Geometry: see drawing. Coordinates: mm, zero at the bounding-box minimum. A direction names the side the tool comes from. Give positions to 0.01 mm unless a question says otherwise; leave off trailing zeros. Write each loop counter-clockwise with the first axis right and the second up, starting at its lowest first coordinate (ties: lowest second). Pieces come first, ordered by that corner, then holes.
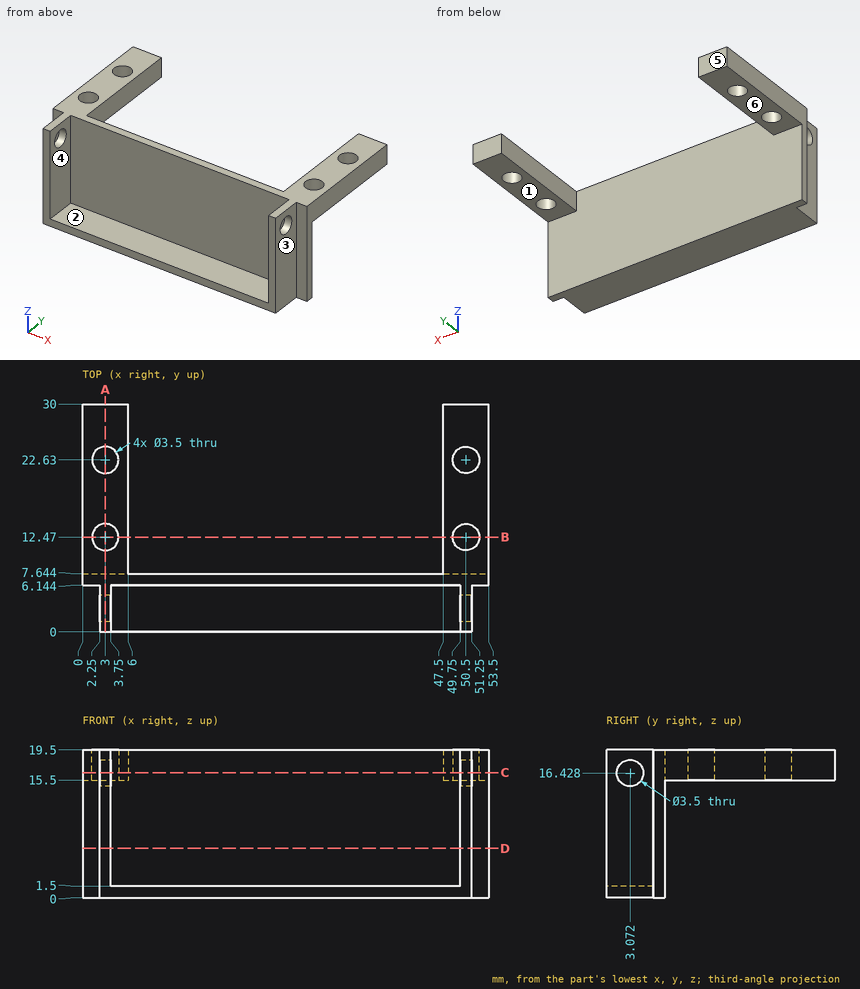
1. Pin query (flat end, axial travel): P1, Ø10, axis at x = 44.5, y = 16, coming from the -Z side; P2, Ø5, axis at y = 3, z = 10.5, coming from the +X side; P3, Ø0.7, axis at x = 52, z = 12.5, coming from the -Y side. Return the tip coordinate at first contact, or that it passes through.
2. Section query A-A (x = 3). Return loops of the section in (y, z).
3. Section query C-C (z = 16.5). Return loops of the section in (x, y).
4. Section query B-B (y = 12.47). Return loops of the section in (x, z).
5. Pull-direction query (X, two-part tool) for the marked faces 1, 2 and 3; classes: pulls with the +X half, pulls with the -X half, needs draft (parallel to the pull), parting line crosses it, or undercut.
6. Access query for the marked faces 4, 5 and 6. Directions: +Z, -Z, +X, -X, +Y, -Y. A direction counts if a zero-diameter tool reaches every point of the face in a straight line with its end or side. Return the directions, or none.
7. Line query: probe 1 along X at (y, z) = (1.5, 5); probe 2 along Y at (x, z) = (3, 17.75); probe 3 along Y at (x, z) = (3, 17.1). Output: solid intervals per line, ascending.
8. Section query D-D (z = 6.5). Return loops of the section in (x, y), plus the area to 3 significant figures.
The answers:
1. P1: stops at z = 15.5
1. P2: stops at x = 51.25
1. P3: stops at y = 6.14
2. outline: (0, 0) - (7.64, 0) - (7.64, 15.5) - (10.72, 15.5) - (10.72, 19.5) - (0, 19.5) - close; (14.22, 15.5) - (20.88, 15.5) - (20.88, 19.5) - (14.22, 19.5) - close; (24.38, 15.5) - (30, 15.5) - (30, 19.5) - (24.38, 19.5) - close; hole circle Ø3.5 at (3.07, 16.43)
3. outline: (0, 6.14) - (2.25, 6.14) - (2.25, 4.82) - (3.75, 4.82) - (3.75, 6.14) - (49.75, 6.14) - (49.75, 4.82) - (51.25, 4.82) - (51.25, 6.14) - (53.5, 6.14) - (53.5, 30) - (47.5, 30) - (47.5, 7.64) - (6, 7.64) - (6, 30) - (0, 30) - close; (2.25, 0) - (3.75, 0) - (3.75, 1.32) - (2.25, 1.32) - close; (49.75, 0) - (51.25, 0) - (51.25, 1.32) - (49.75, 1.32) - close; hole circle Ø3.5 at (3, 12.47); hole circle Ø3.5 at (3, 22.63); hole circle Ø3.5 at (50.5, 12.47); hole circle Ø3.5 at (50.5, 22.63)
4. outline: (0, 15.5) - (1.25, 15.5) - (1.25, 19.5) - (0, 19.5) - close; (4.75, 15.5) - (6, 15.5) - (6, 19.5) - (4.75, 19.5) - close; (47.5, 15.5) - (48.75, 15.5) - (48.75, 19.5) - (47.5, 19.5) - close; (52.25, 15.5) - (53.5, 15.5) - (53.5, 19.5) - (52.25, 19.5) - close
5. face 1: needs draft
5. face 2: undercut
5. face 3: pulls with the +X half
6. face 4: +Z, -Y
6. face 5: +Z, -Z, +X, -X, +Y
6. face 6: -Z, +X, -X, +Y
7. probe 1: x = 2.25 to 3.75, 49.75 to 51.25
7. probe 2: y = 0 to 1.93, 4.22 to 10.72, 14.22 to 20.88, 24.38 to 30
7. probe 3: y = 0 to 1.46, 4.69 to 10.72, 14.22 to 20.88, 24.38 to 30
8. outline: (0, 6.14) - (2.25, 6.14) - (2.25, 0) - (3.75, 0) - (3.75, 6.14) - (49.75, 6.14) - (49.75, 0) - (51.25, 0) - (51.25, 6.14) - (53.5, 6.14) - (53.5, 7.64) - (0, 7.64) - close
8. area: 98.7 mm2
